Autodesk Inventor part; units mm, degrees
ref_plane "fla_XY" through (0, 0, 0) normal (0, 0, 1) x (1, 0, 0)
ref_plane "fla_YZ" through (0, 0, 0) normal (1, 0, 0) x (0, 1, 0)
ref_plane "fla_ZX" through (0, 0, 0) normal (0, 1, 0) x (0, 0, 1)
sketch "Sketch_1" plane through (0, 0, 0) normal (1, 0, 0) x (0, 1, 0)
  line L0 (0, -14.1) -> (0, 0)
  line L1 (34, 0) -> (14, 0)
  line L2 (14, 0) -> (14, -14.1)
  line L3 (14, -14.1) -> (15.75, -14.1)
  line L4 (15.75, -14.1) -> (15.75, -9.1)
  line L5 (15.75, -9.1) -> (34, -9.1)
  line L6 (34, -9.1) -> (34, 0)
revolve "Revolution1" add sketch "Sketch_1" angle 360 about axis through (0, 0, -14.1) along (0, 0, 1)
chamfer "Chamfer1" distance 0.6 distance2 1 1 edges at (0, -15.75, -14.1) measured on face at (1.2564, 15.0141, -14.1)
sketch "Sketch2" plane through (0, 0, 0) normal (0, 0, 1) x (1, 0, 0)
  point P0 (24.1481, -6.4705)
hole "Hole1" at (24.1481, -6.4705, 0) direction (0, 0, -1) diameter 3.242 depth 9.1 counterbore diameter 6 counterbore depth 2.9
pattern_linear "Rectangular Pattern1" count 2 spacing 35.3553 along (-0.5, 0.866, 0) count 2 spacing 35.3553 along (-0.866, -0.5, 0) of "Hole1"
sketch "Sketch3" plane through (0, 0, 0) normal (0, 0, 1) x (1, 0, 0)
  point P0 (17.6777, -17.6777)
hole "Hole2" at (17.6777, -17.6777, 0) direction (0, 0, -1) diameter 6.6 depth 14.1 counterbore diameter 11 counterbore depth 4.6
pattern_linear "Rectangular Pattern2" count 2 spacing 35.3553 along (0, 1, 0) count 2 spacing 35.3553 along (-1, 0, 0) of "Hole2"
sketch "Sketch_6" plane through (0, 0, -9.1) normal (0, 0, 1) x (1, 0, 0)
  arc A0 (-25.5, 3) -> (-25.5, -3) centre (-25.5, 0) ccw
  line L0 (-25.5, -3) -> (-25, -3)
  arc A1 (-25, -3) -> (-25, 3) centre (-25, 0) ccw
  line L1 (-25, 3) -> (-25.5, 3)
extrude "Extrusion1" cut sketch "Sketch_6" along normal blind 5.5
ref_plane "fla_XY" through (0, 0, 0) normal (0, 0, 1) x (1, 0, 0)
ref_plane "fla_YZ" through (0, 0, 0) normal (1, 0, 0) x (0, 1, 0)
ref_plane "fla_ZX" through (0, 0, 0) normal (0, 1, 0) x (0, 0, 1)
properties part number "SCHUNK-1013180-ISO-1-50-M6 Universalflansch Co-act-EGP-C"
The model under review builds one solid part; all positions refer to its coordinate system, in mm. A direction names the side the tool comes from. Round coordinates to 2 decimals unless told otherwise and drop trailing zeros. Order: outer loops, then holes, each group sorted by start corner. A loop starts at its lowest first (then second) coordinate and runs counter-clockwise, first axis right, second up. Notation, with made-up numbers: (80, 76) -> (112, 76) arc R18 ccw to (112, 100) -> close; hole circle Ø8 at (30, -11). An arc over 180 degrees is marked (long way). Write item = value, one per line. Start each with the question number.
Item 1: For faces 1 (the face through (-5.032, -24.896, -6.043)), 2 (the face through (15, 7, -9.1)), 3 (the face through (-22.32, -20.63, -2.33)), list the 3-axis set-ups (+Z, -Z, +X, -X, +Y, -Y) from which the entire face can be reached by the end or side of a thin tool; tool diameter is ignored.
Item 2: Consider section D-D on x = 19. Write out the cut boundary in (y, z), plus the area to 3 significant figures.
Item 3: Clearance check with flat-ended pins moving along their axes: pin 1 Ø1 at (y, z) = (6.5, -7.5) entering from -X; pin 2 Ø17.5 at (x, y) = (-17.68, -17.68) entering from -Z; pin 3 Ø4 at (x, z) = (-12.5, -11.5) entering from -Y; pin 4 Ø3 at (x, y) = (9, 6) entering from +Z. State where each tip first meets the part, or that it passes through.
Item 4: Consider section A-A on x = 0. Write out the cut boundary in (y, z), plus the area to 3 significant figures.
Item 5: For line 1 along Y through (x, z) = (-18.5, -6.25); line 2 along Y through (x, z) = (0, -8.25), list the stretches that pass through material, from the lowest coordinate up.
Item 6: Consider section B-B on y = 0. Write out the cut boundary in (x, z), plus the area to 3 significant figures.
Item 7: Mouldability with a two-part tool opening along X and no side actions: class faces 4 (the face through (-15.616, -2.05, -11.072)), 5 (the face through (-28.5, -0.1, -6.4)), 6 (the face through (10.03, 10.03, -14.1)) as released by +X, released by -X, zero draft, split by the parting line, or undercut.
Item 8: Consider section C-C on z = -7.5. Count the separate pieces of the cut face and the enclosed holes in it, plus the area to 3 significant figures.
Conclusion:
q1.face_1 = +Z, -Z
q1.face_2 = -Z
q1.face_3 = +Z
q2.outline = (-28.2, -9.1) -> (-20.7, -9.1) -> (-20.7, -4.6) -> (-23.02, -4.6) -> (-23.02, 0) -> (-28.2, 0) -> close; (-14.65, -9.1) -> (14.65, -9.1) -> (14.65, -4.6) -> (12.34, -4.6) -> (12.34, 0) -> (-12.34, 0) -> (-12.34, -4.6) -> (-14.65, -4.6) -> close; (20.7, -9.1) -> (28.2, -9.1) -> (28.2, 0) -> (23.02, 0) -> (23.02, -4.6) -> (20.7, -4.6) -> close
q2.area = 361 mm2
q3.pin_1 = -33.47
q3.pin_2 = -9.1
q3.pin_3 = -11.74
q3.pin_4 = through
q4.outline = (-34, -9.1) -> (-15.75, -9.1) -> (-15.75, -13.1) -> (-15.15, -14.1) -> (-14, -14.1) -> (-14, 0) -> (-34, 0) -> close; (14, -14.1) -> (15.15, -14.1) -> (15.75, -13.1) -> (15.75, -9.1) -> (34, -9.1) -> (34, 0) -> (14, 0) -> close
q4.area = 381 mm2
q5.line_1 = -28.53 to -20.87, -14.48 to 14.48, 20.87 to 28.53
q5.line_2 = -34 to -14, 14 to 34
q6.outline = (-34, -9.1) -> (-28.5, -9.1) -> (-28.5, -3.6) -> (-22, -3.6) -> (-22, -9.1) -> (-15.75, -9.1) -> (-15.75, -13.1) -> (-15.15, -14.1) -> (-14, -14.1) -> (-14, 0) -> (-34, 0) -> close; (14, -14.1) -> (15.15, -14.1) -> (15.75, -13.1) -> (15.75, -9.1) -> (34, -9.1) -> (34, 0) -> (14, 0) -> close
q6.area = 345 mm2
q7.face_4 = split by the parting line
q7.face_5 = undercut
q7.face_6 = zero draft
q8.separate_pieces = 1
q8.enclosed_holes = 10
q8.area = 2,810 mm2
